Autodesk Inventor part; units mm, degrees
ref_plane "YZ Plane" through (0, 0, 0) normal (1, 0, 0) x (0, 1, 0)
ref_plane "XZ Plane" through (0, 0, 0) normal (0, 1, 0) x (-1, 0, 0)
ref_plane "XY Plane" through (0, 0, 0) normal (0, 0, 1) x (1, 0, 0)
sketch "スケッチ1" plane through (0, 0, 0) normal (0, 0, 1) x (1, 0, 0)
  circle A0 centre (0, 0) radius 2.5
  circle A1 centre (0, 0) radius 1.8
  dimension "d0" = 5
  dimension "d1" = 3.6
extrude "押し出し1" add sketch "スケッチ1" against normal blind 2.5
sketch "スケッチ2" plane through (0, 0, -2.5) normal (0, 0, -1) x (-1, 0, 0)
  line L0 (-3, 2.5) -> (3, 2.5)
  line L1 (3, 2.5) -> (3, -2.5)
  line L2 (3, -2.5) -> (-3, -2.5)
  line L3 (-3, -2.5) -> (-3, 2.5)
  point P0 (0, 0)
  dimension "d4" = 2.5
  dimension "d5" = 5
  dimension "d6" = 3
  dimension "d7" = 6
extrude "押し出し2" add sketch "スケッチ2" along normal blind 14.5
sketch "スケッチ3" plane through (-3, -2.5, -2.5) normal (0, -1, 0) x (1, 0, 0)
  circle A0 centre (3, -3.6) radius 0.725
  line L0 (3, 0) -> (6, 0)
  circle A1 centre (3, -10.6) radius 0.725
  point P0 (3, 2.5)
  dimension "d10" = 1.45
  dimension "d11" = 3.6
  dimension "d12" = 1.45
  dimension "d13" = 7
extrude "押し出し3" add sketch "スケッチ3" along normal blind 0.8
sketch "スケッチ4" plane through (-3, -2.5, -2.5) normal (0, -1, 0) x (1, 0, 0)
  line L0 (5.35, -2.2) -> (5.55, -2.2)
  line L1 (5.55, -2.2) -> (5.55, -3.2)
  line L2 (5.55, -3.2) -> (5.35, -3.2)
  line L3 (5.35, -3.2) -> (5.35, -2.2)
  line L4 (0.65, -4) -> (0.45, -4)
  line L5 (0.45, -4) -> (0.45, -5)
  line L6 (0.45, -5) -> (0.65, -5)
  line L7 (0.65, -5) -> (0.65, -4)
  circle A0 centre (3, -3.6) radius 0.725
  point P0 (3, 2.5)
  dimension "d16" = 0.2
  dimension "d17" = 0.2
  dimension "d18" = 2.55
  dimension "d19" = 2.55
  dimension "d20" = 1.4
  dimension "d21" = 1.4
  dimension "d22" = 1
  dimension "d23" = 1
extrude "押し出し4" add sketch "スケッチ4" along normal blind 2.4 contours L0 L1 L2 L3 | L7 L6 L5 L4
sketch "スケッチ5" plane through (-3, -2.5, -2.5) normal (0, -1, 0) x (1, 0, 0)
  circle A0 centre (3, -10.6) radius 0.725
  line L0 (5.55, -2.2) -> (5.55, -3.2)
  line L1 (5.55, -3.2) -> (5.35, -3.2)
  line L2 (5.35, -3.2) -> (5.35, -2.2)
  line L3 (5.35, -2.2) -> (5.55, -2.2)
  line L4 (0.65, -4) -> (0.65, -5)
  line L5 (0.65, -5) -> (0.45, -5)
  line L6 (0.45, -5) -> (0.45, -4)
  line L7 (0.45, -4) -> (0.65, -4)
  circle A1 centre (3, -3.6) radius 0.725
  circle A2 centre (3, -10.6) radius 0.725
  line L8 (0, 0) -> (3, 0)
  line L9 (0, 0) -> (0, -14.5)
  line L10 (6, -14.5) -> (0, -14.5)
  line L11 (6, 0) -> (6, -14.5)
  line L12 (3, 0) -> (6, 0)
  line L13 (5.35, -11.3) -> (5.55, -11.3)
  line L14 (5.55, -11.3) -> (5.55, -12.8)
  line L15 (5.55, -12.8) -> (5.35, -12.8)
  line L16 (5.35, -12.8) -> (5.35, -11.3)
  point P0 (3, 2.5)
  dimension "d26" = 0.2
  dimension "d27" = 1.5
  dimension "d28" = 2.2
  dimension "d29" = 2.55
extrude "押し出し5" add sketch "スケッチ5" along normal blind 2.4 contours L13 L14 L15 L16
fillet "フィレット1" radius 0.5 6 edges at (2.45, -4.9, -5.7) (2.45, -4.9, -4.7) (-2.45, -4.9, -6.5) (-2.45, -4.9, -7.5) (2.45, -4.9, -13.8) (2.45, -4.9, -15.3)
properties part number "MJ-4535-3" material "ABS プラスチック"
CAD build for the part. Positions are in the model's coordinates, mm. A direction names the side the tool comes from. Coordinates: 2 decimals unless noted, no trailing zeros. Loops run counter-clockwise (first coordinate to the right, second up) from the corner with the lowest first, then second, coordinate; pieces in that order, holes last. Notation, with made-up numbers: (81, -34) - (127, -34) arc R27 cw to (127, 0) - close; hole circle Ø6 at (57, 41.5). An arc over 180 degrees is marked (long way). Use CSV: the item, a comma, the result in double quotes. Start each with the question number.
Q1. Probe probe 1 along Y at (x, z) = (0, -0.7); probe 2 along Y at (x, z) = (-1.8, -5.25); probe 3 along Z at (x, y) = (-0.2, -1.5). List the from-to ranges inside material, lowest first. Write a range as from..to.
Q2. Drop flat-ended pins along their axis: P1, Ø1.6, axis at x = -0.5, z = -6.5, coming from the -Y side; P2, Ø0.5, axis at y = -4, z = -7, coming from the +X side; P3, Ø0.9, axis at x = 2, y = 0.5, coming from the +Z side; P4, Ø0.8, axis at y = -3.5, z = -14.5, coming from the -X side. Give the stop position or say it passes through.
Q3. Cut at D-D, the plane z = -6.1. List the corners of the cut face in (x, y) (3 decimals), then the cut area to 3 significant figures.
Q4. Cut at B-B, the plane y = 0. List the corners of the cut face in (x, z).
Q5. Two-plate mould, pull along X, no slides. Class faces 5 (the flat face through (2.7, 0.2, -2.5)), 6 (the cylindrical face through (1.717, 0.541, -1.232)), 7 (the flat face through (-3, 0, -10)): +X half, -X half, draft (parallel to the pull), parting line (faces both ways), or undercut.
Q6. Cut at A-A, the plane z = -14.5. List the corners of the cut face in (x, y).
Q7. 3-axis set-ups, long thin cutter, end or side, ignore diameter. For faces 1 (the cylindrical face through (-0.54, -2.44, -1.23)), 2 (the cylindrical face through (-0.09, -2.89, -13.82)), 3 (the flat face through (2.55, -4, -15)), 4 (the flat face through (-2.7, -0.2, -2.5)): which of +Z, -Z, +X, -X, +Y, -Y reach the whole face in a straight line?
Here are the results:
1,probe 1,"-2.5..-1.8, 1.8..2.5"
1,probe 2,"-2.5..2.5"
1,probe 3,"-17..-2.5"
2,P1,"y = -3.3"
2,P2,"x = -2.35"
2,P3,"z = 0"
2,P4,"x = 2.35"
3,outline,"(-3, -2.5) - (-0.725, -2.5) - (-0.725, -3.3) - (0.725, -3.3) - (0.725, -2.5) - (3, -2.5) - (3, 2.5) - (-3, 2.5) - close"
3,area,"31.2 mm2"
4,outline,"(-3, -17) - (3, -17) - (3, -2.5) - (2.5, -2.5) - (2.5, 0) - (1.8, 0) - (1.8, -2.5) - (-1.8, -2.5) - (-1.8, 0) - (-2.5, 0) - (-2.5, -2.5) - (-3, -2.5) - close"
5,face 5,"draft"
5,face 6,"undercut"
5,face 7,"-X half"
6,outline,"(-3, -2.5) - (2.35, -2.5) - (2.35, -4.9) - (2.55, -4.9) - (2.55, -2.5) - (3, -2.5) - (3, 2.5) - (-3, 2.5) - close"
7,face 1,"+Z"
7,face 2,"-Y"
7,face 3,"+Z, -Z, +X, -Y"
7,face 4,"+Z, -X"
